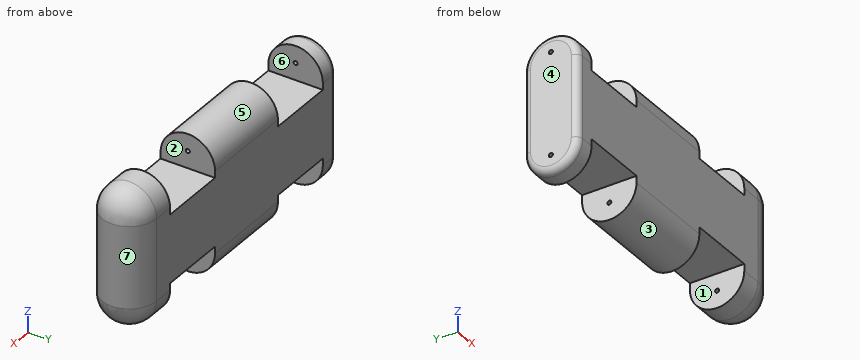
```python
from build123d import *

# Parameters (mm, degrees)
BOSS_EXTRUDE1_DEPTH     = 40
CUT_EXTRUDE1_DEPTH      = 291.688837075
CUT_EXTRUDE1_DEPTH_BACK = 291.688837075
SKETCH2_R               = 3
CUT_EXTRUDE2_DEPTH      = 291.688837075
CUT_EXTRUDE2_DEPTH_BACK = 291.688837075
SKETCH3_R               = 3
CUT_EXTRUDE3_DEPTH      = 415.246303544
CUT_EXTRUDE3_DEPTH_BACK = 415.246303544
CUT_EXTRUDE4_DEPTH      = 415.246303544
CUT_EXTRUDE4_DEPTH_BACK = 415.246303544
BOSS_EXTRUDE3_DEPTH     = 60
REVOLVE1_ANGLE          = 90
FILLET1_R               = 10


with BuildPart() as part:
    # Sketch1 → Boss-Extrude1 (new, symmetric)
    with BuildSketch(Plane(origin=(0, 0, 0), x_dir=(1, 0, 0), z_dir=(0, 1, 0))):
        Polygon((-200, 100), (-170, 100), (-170, 50), (-70, 50), (-70, 100), (70, 100), (70, 50), (170, 50), (170, 100), (200, 100), (200, -100), (170, -100), (170, -50), (70, -50), (70, -100), (-70, -100), (-70, -50), (-170, -50), (-170, -100), (-200, -100), align=None)
    extrude(amount=BOSS_EXTRUDE1_DEPTH, both=True)

    # Sketch2 → Cut-Extrude1 (cut, two sides: drawn at the far end of the back side and taken through both)
    with BuildSketch(Plane.ZY.offset(70).offset(-CUT_EXTRUDE1_DEPTH_BACK)):
        with Locations((-75, 0)):
            Circle(SKETCH2_R)
    extrude(amount=CUT_EXTRUDE1_DEPTH + CUT_EXTRUDE1_DEPTH_BACK, mode=Mode.SUBTRACT)

    # Sketch3 → Cut-Extrude2 (cut, two sides: drawn at the far end of the back side and taken through both)
    with BuildSketch(Plane.ZY.offset(70).offset(-CUT_EXTRUDE2_DEPTH_BACK)):
        with Locations((75, 0)):
            Circle(SKETCH3_R)
    extrude(amount=CUT_EXTRUDE2_DEPTH + CUT_EXTRUDE2_DEPTH_BACK, mode=Mode.SUBTRACT)

    # Sketch4 → Cut-Extrude3 (cut, two sides: drawn at the far end of the back side and taken through both)
    with BuildSketch(Plane.ZY.offset(200).offset(-CUT_EXTRUDE3_DEPTH_BACK)):
        with BuildLine():
            Line((-60, -40), (-60, -70.289993794))
            Line((-60, -70.289993794), (-136.864216991, -70.289993794))
            Line((-136.864216991, -70.289993794), (-136.864216991, 63.942219024))
            Line((-136.864216991, 63.942219024), (-60, 63.942219024))
            Line((-60, 63.942219024), (-60, 40))
            ThreePointArc((-60, 40), (-100, 0), (-60, -40))
        make_face()
    extrude(amount=CUT_EXTRUDE3_DEPTH + CUT_EXTRUDE3_DEPTH_BACK, mode=Mode.SUBTRACT)

    # Sketch5 → Cut-Extrude4 (cut, two sides: drawn at the far end of the back side and taken through both)
    with BuildSketch(Plane.ZY.offset(200).offset(-CUT_EXTRUDE4_DEPTH_BACK)):
        with BuildLine():
            Line((60, -40), (60, -76.328121014))
            Line((60, -76.328121014), (141.05428579, -76.328121014))
            Line((141.05428579, -76.328121014), (141.05428579, 68.89657982))
            Line((141.05428579, 68.89657982), (60, 68.89657982))
            Line((60, 68.89657982), (60, 40))
            ThreePointArc((60, 40), (100, 0), (60, -40))
        make_face()
    extrude(amount=CUT_EXTRUDE4_DEPTH + CUT_EXTRUDE4_DEPTH_BACK, mode=Mode.SUBTRACT)

    # Sketch7 → Boss-Extrude3 (add, symmetric)
    with BuildSketch(Plane.XY):
        with BuildLine():
            Line((200, 40), (200, -40))
            ThreePointArc((200, -40), (240, 0), (200, 40))
        make_face()
    extrude(amount=BOSS_EXTRUDE3_DEPTH, both=True)

    # Sketch8 → Revolve1 (revolve)
    with BuildSketch(Plane.XY.offset(60)):
        with BuildLine():
            Line((200, 40), (200, -40))
            ThreePointArc((200, -40), (240, 0), (200, 40))
        make_face()
    revolve1 = revolve(axis=Axis((200, 40, 60), (0, -1, 0)), revolution_arc=REVOLVE1_ANGLE)

    # Mirror1: Revolve1 across plane
    add(revolve1.mirror(Plane.XY))

    # Fillet1
    fillet1_edges = [part.edges().sort_by_distance(p)[0] for p in [
        (-200, 0, 100),
        (-200, -40, 0),
        (-200, 40, 0),
        (-200, 0, -100),
    ]]
    fillet(fillet1_edges, radius=FILLET1_R)


solid = part.part
```
Could you check a few things on this model? Use its own coordinates, in mm. Face numbers are marked on the shaded views. A direction names the side the tool comes from. Coordinates: 2 decimals unless noted, no trailing zeros. Order: outer loops, then holes, each group sorted by start corner. A loop starts at its lowest first (then second) coordinate and runs counter-clockwise, first axis right, second up. Notation, with made-up numbers: M 55,10.25 L 110,10.25 A36 ccw 110,46.25 Z; hole C 59,66 d6. An arc over 180 degrees is marked long. Use a Markdown table: item, result. Add a question column.
Q1. Which directions (+Z, -Z, +X, -X, +Y, -Y) give clear straight access to the entire face, cutting with the end or side of a thin tool? Please do the marked faces 1, 2 and 3.
Q2. I want a section at A-A on x = -55. List the corners of the cut face in (y, z) for me.
Q3. I'm going to push flat-ended pins straight in: pin 1 (8 mm diameter, centred on y = 25.5, z = 45, fed in from +X); pin 2 (5.5 mm diameter, centred on y = 0, z = -75, fed in from +X); pin 3 (1.5 mm diameter, centred on x = 192.5, y = -18.5, fed in from +Z). Where does each tip first touch, or does it pass through?
Q4. If I drill on L1, parallel to Z at x = -187, y = 0; L2, parallel to X at y = -3, z = 80; L3, parallel to X at y = -15, z = -80.5, over which ranges is the centre line in solid material (lowest first)?
Q5. I want a section at B-B on z = 83. Give the number of separate pieces and of enclosed holes in the cut face, then the cut area to 3 significant figures.
Q6. I want a section at D-D on z = 10. List the corners of the cut face in (x, y) for me, then the cut area to 3 significant figures.
Q7. We'd pull the mould along X, two halves only. Please class the marked faces 4, 5, 6 and 7: pulls with the +X half, pulls with the -X half, needs draft (parallel to the pull), parting line crosses it, or undercut.
Q8. I want a section at C-C on x = -135.5. List the corners of the cut face in (y, z) for me.
Checked values:
| question | item | result |
|---|---|---|
| 1 | face 1 | -Z, +Y, -Y |
| 1 | face 2 | +Z, +Y, -Y |
| 1 | face 3 | -Z, +X, -X |
| 2 | outline | M -40,-60 A40 ccw 40,-60 L 40,60 A40 ccw -40,60 Z; hole C 0,-75 d6; hole C 0,75 d6 |
| 3 | pin 1 | x = 233.73 |
| 3 | pin 2 | x = 238.08 |
| 3 | pin 3 | z = 95.85 |
| 4 | L1 | -100 to -78, -72 to 72, 78 to 100 |
| 4 | L2 | -200 to -170, -70 to 70, 170 to 234.51 |
| 4 | L3 | -200 to -170, -70 to 70, 170 to 230.9 |
| 5 | separate pieces | 3 |
| 5 | enclosed holes | 0 |
| 5 | area | 14,700 mm² |
| 6 | outline | M -200,-30 A10 ccw -190,-40 L 200,-40 A40 ccw 200,40 L -190,40 A10 ccw -200,30 Z |
| 6 | area | 34,500 mm² |
| 7 | face 4 | pulls with the -X half |
| 7 | face 5 | needs draft |
| 7 | face 6 | undercut |
| 7 | face 7 | pulls with the +X half |
| 8 | outline | M -40,-50 L 40,-50 L 40,50 L -40,50 Z |
